```python
from build123d import *

# Parameters (mm, degrees)
SKETCH1_R           = 1.25
BOSS_EXTRUDE1_DEPTH = 3


with BuildPart() as part:
    # Sketch1 → Boss-Extrude1 (new body)
    with BuildSketch(Plane(origin=(0, 0, 0), x_dir=(1, 0, 0), z_dir=(0, 1, 0))):
        with BuildLine():
            Line((6.30223182, -4.135535586), (6.632271605, -3.805495802))
            ThreePointArc((6.632271605, -3.805495802), (7.850711529, -2.042416999), (8.5, 0))
            ThreePointArc((8.5, 0), (6.01040764, 6.01040764), (0, 8.5))
            ThreePointArc((0, 8.5), (-2.042416999, 7.850711529), (-3.805495802, 6.632271605))
            Line((-3.805495802, 6.632271605), (-4.135535586, 6.30223182))
            Line((-4.135535586, 6.30223182), (-6.30223182, 4.135535586))
            Line((-6.30223182, 4.135535586), (-6.632271605, 3.805495802))
            ThreePointArc((-6.632271605, 3.805495802), (-7.850711529, 2.042416999), (-8.5, 0))
            ThreePointArc((-8.5, 0), (-6.01040764, -6.01040764), (0, -8.5))
            ThreePointArc((0, -8.5), (2.042416999, -7.850711529), (3.805495802, -6.632271605))
            Line((3.805495802, -6.632271605), (4.135535586, -6.30223182))
            Line((4.135535586, -6.30223182), (6.30223182, -4.135535586))
        make_face()
        Circle(SKETCH1_R, mode=Mode.SUBTRACT)
    extrude(amount=BOSS_EXTRUDE1_DEPTH)


solid = part.part
```
The listing builds one solid part. Answer for the finished solid, in the listing's coordinates (mm). Give positions to 0.01 mm unless a question says otherwise; leave off trailing zeros. Order: outer loops, then holes, each group sorted by start corner. A loop starts at its lowest first (then second) coordinate and runs counter-clockwise, first axis right, second up.
1) Find section A-A on y = 1.1. Write down the section's boundary in (x, z), then the cut area to 3 significant figures.
Reported:
outline: (-8.5, 0) arc R7.24 ccw to (-6.63, -3.81) - (-3.81, -6.63) arc R7.24 ccw to (0, -8.5) arc R8.5 ccw to (8.5, 0) arc R7.24 ccw to (6.63, 3.81) - (3.81, 6.63) arc R7.24 ccw to (0, 8.5) arc R8.5 ccw to start; hole circle Ø2.5 at (0, 0)
area: 206 mm2
2) Consider line 1 along X through (y, z) = (1.6, -0.5); line 2 along Z through (x, y) = (-0.75, 2.85); line 3 along Z through (x, y) = (-3.5, 0.65). Determine where each line is inside the solid, lowest interval first.
Reported:
line 1: x = -8.4 to -1.15, 1.15 to 8.49
line 2: z = -8.34 to -1, 1 to 8.47
line 3: z = -6.9 to 7.75
3) Find section B-B on x = 7.75. Write down the section's boundary in (y, z), then the cut area to 3 significant figures.
Reported:
outline: (0, -3.49) - (3, -3.49) - (3, 2.24) - (0, 2.24) - close
area: 17.2 mm2
4) Find section C-C on z = 2.5. Write down the section's boundary in (x, y), then the cut area to 3 significant figures.
Reported:
outline: (-8.12, 0) - (7.61, 0) - (7.61, 3) - (-8.12, 3) - close
area: 47.2 mm2
5) Given P1, Ø6, axis at x = -5, z = -0.5, coming from the -Y side; P2, Ø1.5, axis at x = 0, z = 0, coming from the +Y side; P3, Ø1, axis at x = -5.5, y = 2, coming from the -Z side; P4, Ø1.5, axis at x = 2.5, y = 1.5, coming from the +Z side, each flat-ended and moving along its own axis, determine where each tip first touches the part or whether it passes through.
Reported:
P1: stops at y = 0
P2: passes through
P3: stops at z = -5.44
P4: stops at z = 7.99
6) Determine the mould class of faces 1 (the face through (2, 0, 0)), 2 (the face through (-2.02, 1.48, -7.86)), 3 (the face through (-0.27, 1.48, 1.22)) for opening direction Z: pulls with the +Z half, pulls with the -Z half, needs draft (parallel to the pull), parting line crosses it, or undercut.
Reported:
face 1: needs draft
face 2: pulls with the -Z half
face 3: undercut
